Design review of the part built by this model. Coordinates are the model's own, in mm. Face numbers are marked on the shaded views. A direction names the side the tool comes from. Round coordinates to 2 decimals unless told otherwise and drop trailing zeros. Loops run counter-clockwise (first coordinate to the right, second up) from the corner with the lowest first, then second, coordinate; pieces in that order, holes last. Notation, with made-up numbers: M -20.5,4 L -0.5,4 A26 ccw -0.5,26 Z; hole C 47.5,52.25 d1. An arc over 180 degrees is marked long. Use a Markdown table: item, result.
from build123d import *

# Parameters (mm, degrees)
EXTRUDE_1_DEPTH     = 8
SKETCH_2_R          = 10
EXTRUDE_2_DEPTH     = 8
SKETCH_3_W          = 19.850439241
SKETCH_3_H          = 8
EXTRUDE_3_DEPTH     = 3
SKETCH_4_R          = 1.8
CUT_EXTRUDE_1_DEPTH = 5


with BuildPart() as part:
    # Sketch 1 → Extrude 1 (new body)
    with BuildSketch(Plane.XY):
        with BuildLine():
            Line((-23, 0), (-23, -40.29))
            Line((-23, -40.29), (23, -40.29))
            Line((23, -40.29), (23, 0))
            ThreePointArc((23, 0), (0, 23), (-23, 0))
        make_face()
    extrude(amount=EXTRUDE_1_DEPTH)

    # Sketch 2 → Extrude 2 (add)
    with BuildSketch(Plane.XY.offset(8)):
        Circle(SKETCH_2_R)
    extrude(amount=EXTRUDE_2_DEPTH)

    # Sketch 3 → Extrude 3 (add)
    with BuildSketch(Plane(origin=(0, -40.29, 0), x_dir=(-1, 0, 0), z_dir=(0, -1, 0))):
        with Locations((-0.065968244, -4)):
            Rectangle(SKETCH_3_W, SKETCH_3_H)
    extrude(amount=EXTRUDE_3_DEPTH)

    # Sketch 4 → Cut-Extrude 1 (cut)
    with BuildSketch(Plane(origin=(0, -40.29, 0), x_dir=(-1, 0, 0), z_dir=(0, -1, 0))):
        with Locations(Location((19, -4, 0), (0, 0, 90))):
            Circle(SKETCH_4_R)
    cut_extrude_1 = extrude(amount=-CUT_EXTRUDE_1_DEPTH, mode=Mode.SUBTRACT)

    # Mirror 1: Cut-Extrude 1 across plane
    add(cut_extrude_1.mirror(Plane.ZY), mode=Mode.SUBTRACT)


solid = part.part
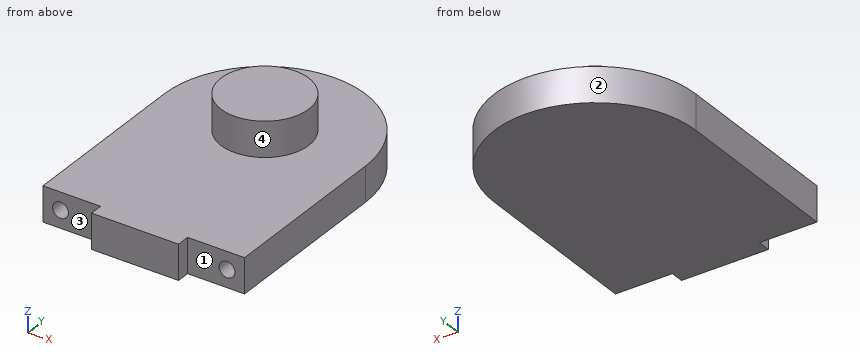
1. Machinability: for the marked faces 1, 2, 3 and 4, which of the approach directions +Z, -Z, +X, -X, +Y, -Y give a long, thin tool a straight path to every point of the face, cutting with its end or side? Answer none if there is none.
Check values:
| item | result |
|---|---|
| face 1 | +Z, -Z, +X, -Y |
| face 2 | +Z, -Z, +Y |
| face 3 | +Z, -Z, -X, -Y |
| face 4 | +Z |
2. Take a section at C-C on y = -31. Give the boundary of the cut face in (x, z), and give its area (3 significant figures).
Check values:
| item | result |
|---|---|
| outline | M -23,0 L 23,0 L 23,8 L -23,8 Z |
| area | 368 mm² |
3. Insertion check: pin 1 (3 mm diameter, centred on x = -8.5, z = 8.5, fed in from +Y); pin 2 (4 mm diameter, centred on x = -13.5, z = 5, fed in from -Y); pin 3 (6 mm diameter, centred on y = 6, z = 8, fed in from +X). Each pin has a flat end and moves straight along its axis. Give the tip position at first contact, or say it passes through.
Check values:
| item | result |
|---|---|
| pin 1 | stops at y = 21.88 |
| pin 2 | stops at y = -40.29 |
| pin 3 | stops at x = 22.8 |
4. Take a section at A-A on z = 7.25. Give the boundary of the cut face in (x, y).
Check values:
| item | result |
|---|---|
| outline | M -23,-40.29 L -9.86,-40.29 L -9.86,-43.29 L 9.99,-43.29 L 9.99,-40.29 L 23,-40.29 L 23,0 A23 ccw -23,0 Z |
5. Take a section at D-D on z = 4. Give the boundary of the cut face in (x, y), and give its area (3 significant figures).
Check values:
| item | result |
|---|---|
| outline | M -23,-40.29 L -20.8,-40.29 L -20.8,-35.29 L -17.2,-35.29 L -17.2,-40.29 L -9.86,-40.29 L -9.86,-43.29 L 9.99,-43.29 L 9.99,-40.29 L 17.2,-40.29 L 17.2,-35.29 L 20.8,-35.29 L 20.8,-40.29 L 23,-40.29 L 23,0 A23 ccw -23,0 Z |
| area | 2,710 mm² |
6. Take a section at B-B on x = 0. Give the boundary of the cut face in (y, z), and give its area (3 significant figures).
Check values:
| item | result |
|---|---|
| outline | M -43.29,0 L 23,0 L 23,8 L 10,8 L 10,16 L -10,16 L -10,8 L -43.29,8 Z |
| area | 690 mm² |
7. Wall thickness on line 1 along X through (y, z) = (-36.6, 4); line 2 along Z through (x, y) = (19, -38.5); line 3 along Z through (x, y) = (-9.5, -18.5): over which ranges is each line inside the solid? List them lowest first. Write a range as from..to.
Check values:
| item | result |
|---|---|
| line 1 | x = -23..-20.8, -17.2..17.2, 20.8..23 |
| line 2 | z = 0..2.2, 5.8..8 |
| line 3 | z = 0..8 |
